Check sheet for the drawn part. Datum: minimum x, y, z corner. Units: mm. Give positions to 0.01 mm unless a question says otherwise; leave off trailing zeros. Order: outer loops, then holes, each group sorted by start corner. A loop starts at its lowest first (then second) coordinate and runs counter-clockwise, first axis right, second up. Notation, with made-up numbers: M 35,39.25 L 79,39.25 A31 ccw 79,63.25 Z; hole C 76,-30 d6. An arc over 180 degrees is marked long. Answer as CSV lines item,"result". Start each with the question number.
Q1. Section check A-A, the plane z = 35. Record the boundary of the cut face in (x, y).
Q2. Section check C-C, the plane y = 1. Count the separate pieces of the cut face and the enclosed holes in it, then the cut area to 3 significant figures.
Q3. Go/stop test with a flat-tipped pin: pin 1 (4 mm diameter, centred on x = 3, z = 35, fed in from +Y). Record where the tip stops, or that it passes through.
Q4. Thickness scan on line 1 (Z direction, x = 3, y = 0.8); line 2 (X direction, y = 0.7, z = 35); line 3 (X direction, y = 1.45, z = 4). Record the ranges inside material, lowest first.
Q5. Section check B-B, the plane x = 3. Record the boundary of the cut face in (y, z), then the cut area to 3 significant figures.
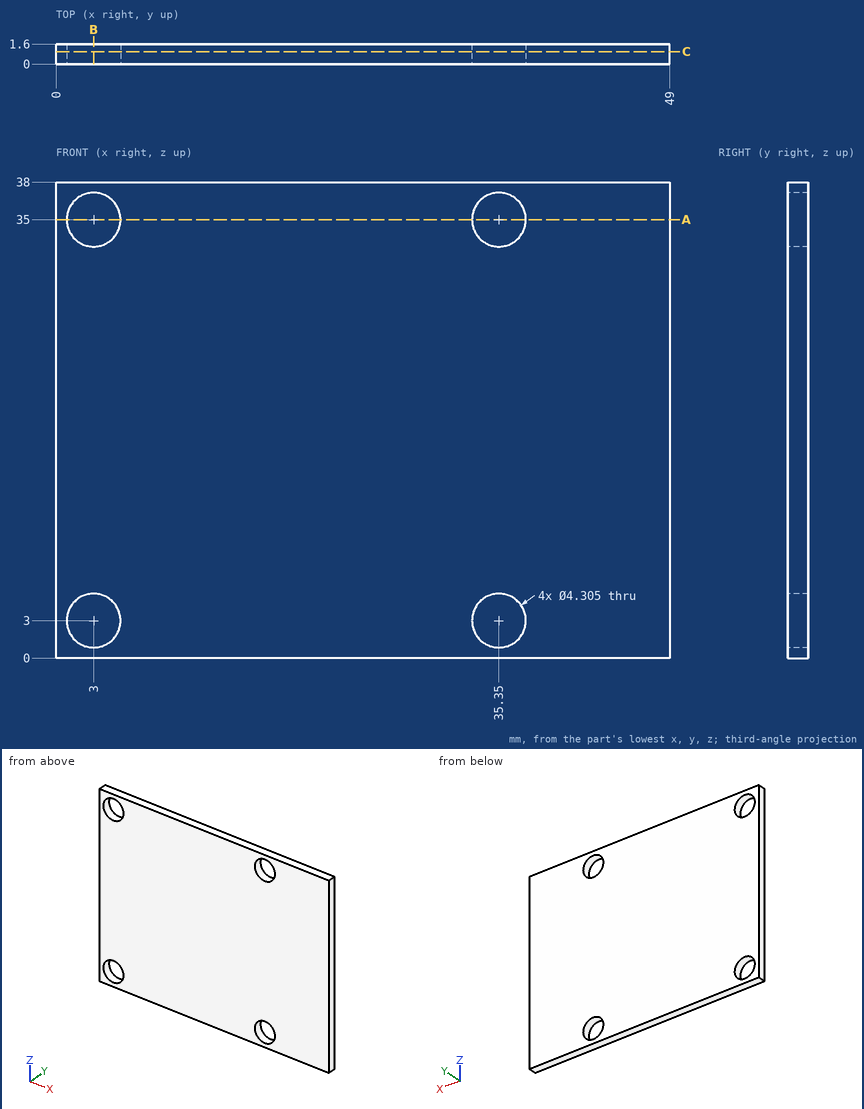
Answer block:
1,outline,"M 0,0 L 0.85,0 L 0.85,1.6 L 0,1.6 Z; M 5.15,0 L 33.2,0 L 33.2,1.6 L 5.15,1.6 Z; M 37.5,0 L 49,0 L 49,1.6 L 37.5,1.6 Z"
2,separate pieces,"1"
2,enclosed holes,"4"
2,area,"1,800 mm2"
3,pin 1,"passes through"
4,line 1,"z = 0 to 0.85, 5.15 to 32.85, 37.15 to 38"
4,line 2,"x = 0 to 0.85, 5.15 to 33.2, 37.5 to 49"
4,line 3,"x = 0 to 1.09, 4.91 to 33.44, 37.26 to 49"
5,outline,"M 0,0 L 1.6,0 L 1.6,0.85 L 0,0.85 Z; M 0,5.15 L 1.6,5.15 L 1.6,32.85 L 0,32.85 Z; M 0,37.15 L 1.6,37.15 L 1.6,38 L 0,38 Z"
5,area,"47.0 mm2"
